For this review, use the dimensioned drawing (mm, ordinates from the lowest corner) and the shaded views. Coordinates: 2 decimals unless noted, no trailing zeros. Order: outer loops, then holes, each group sorted by start corner. A loop starts at its lowest first (then second) coordinate and runs counter-clockwise, first axis right, second up. Notation, with made-up numbers: (69, 17) -> (80, 17) arc R16 ccw to (80, 38) -> close; hole circle Ø10 at (-14.5, 24.25). An arc over 180 degrees is marked (long way). Return JSON: item names as keys, results as strings. Group by question number.
Item 1: For line 1 along Y through (x, z) = (25, 5.75); line 2 along X through (y, z) = (283, 3.25); line 3 along Y through (x, z) = (28, 2), list the stretches that pass through material, from the lowest coordinate up.
Item 2: Take a section at B-B (y = 25). Write out the cut boundary in (x, z).
Item 3: Take a section at A-A (x = 25). Write out the cut boundary in (y, z), then the cut area to 3 significant figures.
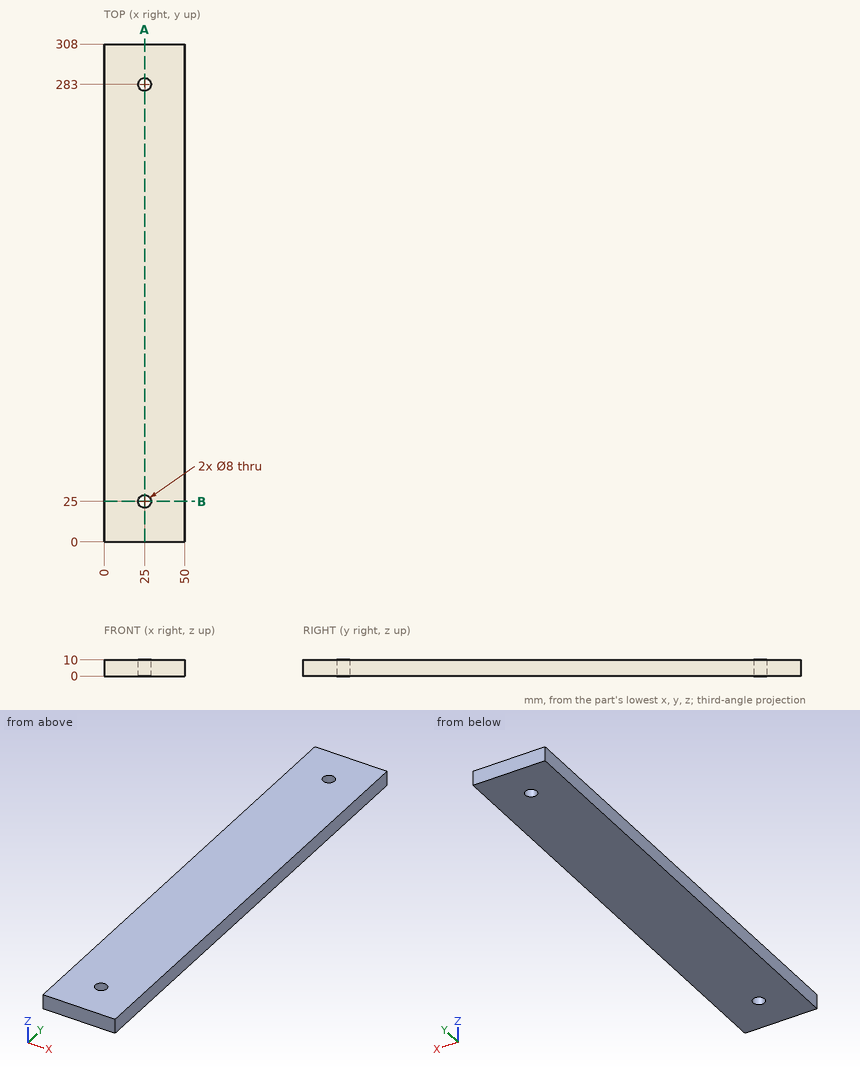
Findings below:
{
 "1": {"line 1": "y = 0 to 21, 29 to 279, 287 to 308", "line 2": "x = 0 to 21, 29 to 50", "line 3": "y = 0 to 22.35, 27.65 to 280.35, 285.65 to 308"},
 "2": {"outline": "(0, 0) -> (21, 0) -> (21, 10) -> (0, 10) -> close; (29, 0) -> (50, 0) -> (50, 10) -> (29, 10) -> close"},
 "3": {"outline": "(0, 0) -> (21, 0) -> (21, 10) -> (0, 10) -> close; (29, 0) -> (279, 0) -> (279, 10) -> (29, 10) -> close; (287, 0) -> (308, 0) -> (308, 10) -> (287, 10) -> close", "area": "2,920 mm2"}
}
